Could you check a few things on this model? Use its own coordinates, in mm. A direction names the side the tool comes from. Give positions to 0.01 mm unless a question says otherwise; leave off trailing zeros. Order: outer loops, then holes, each group sorted by start corner. A loop starts at its lowest first (then second) coordinate and runs counter-clockwise, first axis right, second up. Notation, with made-up numbers: (-1, 53) - (39, 53) arc R32 cw to (39, 87) - close; hole circle Ø6 at (-5.5, 59). An arc over 180 degrees is marked (long way). Put each result on its own line as item: value.
from build123d import *

# Parameters (mm, degrees)
CHANFREIN1_SIZE = 0.5


with BuildPart() as part:
    # Esquisse1 → Révolution1 (revolve)
    with BuildSketch(Plane.XY):
        Polygon((0, 0), (0, 3), (2.4, 3), (2.4, 2.5), (4.4, 2.5), (4.4, 3), (7.4, 3), (7.4, 2), (11, 2), (11, 0), align=None)
    revolve(axis=Axis((11, 0, 0), (-1, 0, 0)))

    # Chanfrein1
    chanfrein1_edges = [part.edges().sort_by_distance(p)[0] for p in [
        (0, -3, 0),
    ]]
    chamfer(chanfrein1_edges, length=CHANFREIN1_SIZE)


solid = part.part
1) We'd pull the mould along X, two halves only. Please class faces 4 (the flat face through (4.4, 2, -2)), 5 (the flat face through (11, 0, 0)), 6 (the flat face through (2.4, -2, -2)), 7 (the flat face through (0, 0, 0)): pulls with the +X half, pulls with the -X half, needs draft (parallel to the pull), parting line crosses it, or undercut.
Filled in:
face 4: undercut
face 5: pulls with the +X half
face 6: undercut
face 7: pulls with the -X half
2) Suppose I cut it at C-C, the plane x = 5.5. List the corners of the cut face in (y, z) for me.
Filled in:
outline: circle Ø6 at (0, 0)
3) I'm going to push flat-ended pins straight in: pin 1 (2 mm diameter, centred on x = 7, z = -1.5, fed in from -Y); pin 2 (1.5 mm diameter, centred on x = 9.5, z = 1.5, fed in from -Y); pin 3 (3 mm diameter, centred on x = 9.5, y = -1, fed in from +Z). Where does each tip first touch, or does it pass through?
Filled in:
pin 1: stops at y = -2.96
pin 2: stops at y = -1.85
pin 3: stops at z = 2
4) Suppose I cut it at A-A, the plane y = 0. List the corners of the cut face in (x, z) for me, and give its area (4 significant figures).
Filled in:
outline: (0, -2.5) - (0.5, -3) - (2.4, -3) - (2.4, -2.5) - (4.4, -2.5) - (4.4, -3) - (7.4, -3) - (7.4, -2) - (11, -2) - (11, 2) - (7.4, 2) - (7.4, 3) - (4.4, 3) - (4.4, 2.5) - (2.4, 2.5) - (2.4, 3) - (0.5, 3) - (0, 2.5) - close
area: 56.55 mm^2
5) Which directions (+Z, -Z, +X, -X, +Y, -Y) give clear straight access to the entire face, cutting with the end or side of a thin tool? Please do faces 1 (the flat face through (7.4, 1, 2)), 2 (the cylindrical face through (3.41, -0.54, 2.44)), 3 (the cylindrical face through (6, -3, 0)).
Filled in:
face 1: +X
face 2: none
face 3: +X, -X
6) If I drill on line 1 (X direction, y = -0.95, z = -2.4); line 2 (X direction, y = -1.8, z = -1.5); line 3 (Y direction, x = 9.5, z = 0.95), over which ranges is the centre line in solid material (lowest first)? Write a range as [from, to].
Filled in:
line 1: x = [0.08, 2.4], [4.4, 7.4]
line 2: x = [0, 7.4]
line 3: y = [-1.76, 1.76]
